The model under review builds one solid part; all positions refer to its coordinate system, in mm. A direction names the side the tool comes from. Give positions to 0.01 mm unless a question says otherwise; leave off trailing zeros. Loops run counter-clockwise (first coordinate to the right, second up) from the corner with the lowest first, then second, coordinate; pieces in that order, holes last. Notation, with made-up numbers: (4, 44) - (25, 44) arc R18 cw to (25, 69) - close; hole circle Ø9 at (74, 1.25). An arc over 180 degrees is marked (long way). Return JSON: item names as keys, results as strings. Group by question number.
from build123d import *

# Parameters (mm, degrees)
SKETCH1_R           = 17.5
SKETCH1_R_2         = 1.5
BOSS_EXTRUDE1_DEPTH = 4
SKETCH3_W           = 12
SKETCH3_H           = 17
SKETCH3_W_2         = 10
SKETCH3_H_2         = 15
BOSS_EXTRUDE2_DEPTH = 10
FILLET1_R           = 2


with BuildPart() as part:
    # Sketch1 → Boss-Extrude1 (new body)
    with BuildSketch(Plane(origin=(0, 0, 0), x_dir=(1, 0, 0), z_dir=(0, 1, 0))):
        with Locations(Location((0, 0, 0), (0, 0, 270))):
            Circle(SKETCH1_R)
        with Locations(Location((12, 6, 0), (0, 0, 270))):
            Circle(SKETCH1_R_2, mode=Mode.SUBTRACT)
        with Locations(Location((12, -6, 0), (0, 0, 270))):
            Circle(SKETCH1_R_2, mode=Mode.SUBTRACT)
        with Locations(Location((-12, 6, 0), (0, 0, 270))):
            Circle(SKETCH1_R_2, mode=Mode.SUBTRACT)
        with Locations(Location((-12, -6, 0), (0, 0, 270))):
            Circle(SKETCH1_R_2, mode=Mode.SUBTRACT)
        with Locations(Location((6, 12, 0), (0, 0, 270))):
            Circle(SKETCH1_R_2, mode=Mode.SUBTRACT)
        with Locations(Location((6, -12, 0), (0, 0, 270))):
            Circle(SKETCH1_R_2, mode=Mode.SUBTRACT)
        with Locations(Location((-6, -12, 0), (0, 0, 270))):
            Circle(SKETCH1_R_2, mode=Mode.SUBTRACT)
        with Locations(Location((-6, 12, 0), (0, 0, 270))):
            Circle(SKETCH1_R_2, mode=Mode.SUBTRACT)
    extrude(amount=BOSS_EXTRUDE1_DEPTH)

    # Sketch3 → Boss-Extrude2 (add)
    with BuildSketch(Plane(origin=(0, 4, 0), x_dir=(1, 0, 0), z_dir=(0, 1, 0))):
        Rectangle(SKETCH3_W, SKETCH3_H)
        Rectangle(SKETCH3_W_2, SKETCH3_H_2, mode=Mode.SUBTRACT)
    extrude(amount=BOSS_EXTRUDE2_DEPTH)

    # Fillet1
    fillet1_edges = [part.edges().sort_by_distance(p)[0] for p in [
        (-6, 4, 0),
        (0, 4, 8.5),
        (6, 4, 0),
        (0, 4, -8.5),
    ]]
    fillet(fillet1_edges, radius=FILLET1_R - 0.0001)  # a hair under: the kernel refuses the full size


solid = part.part
Item 1: For L1, parallel to X at y = 8.5, z = 1.5; L2, parallel to X at y = 2.2, z = 6; L3, parallel to X at y = 1, z = -12, list the stretches that pass through material, from the lowest coordinate up. Write a range as from..to.
Item 2: Take a section at B-B (x = 7). State the section outline as (y, z) points.
Item 3: Mouldability with a two-part tool opening along X and no side actions: class faces 6 (the face through (0, 0, 0)), 7 (the face through (12.07, 1.97, 4.5)), 8 (the face through (-10.648, 1.972, -13.887)) as +X half, -X half, draft (parallel to the pull), parting line (faces both ways), or undercut.
Item 4: Take a section at C-C (z = -12). State the section outline as (x, y) points.
Item 5: Tool access review of faces 1 (the face through (-5.93, 1.97, -13.5)), 2 (the face through (0, 4, 11)), 3 (the face through (-6, 10, 0)), 4 (the face through (0.11, 4.57, 9.1)), 5 (the face through (6, 10, 0)): name each direction out of +Z, -Z, +X, -X, +Y, -Y from which nothing blocks a thin tool from reaching the whole face with its end or side.
Item 6: For P1, Ø6.5, axis at y = 9, z = -2.5, coming from the -X side; P2, Ø4, axis at x = -12, z = 6, coming from the -Y side; P3, Ø4, axis at y = 7.5, z = -5.5, coming from the +X side; P4, Ø2, axis at x = 7.5, y = 10, coming from the -Z side, all flat-tipped, find the tip position at first contact; note any pin that passes through.
Item 7: Take a section at A-A (y = 12.75). State the section outline as (x, z) points.
Item 8: Take a section at D-D (x = 0). State the section outline as (y, z) points, then the cut area to 3 significant figures.
Check sheet entries:
{
 "1": {"L1": "x = -6..-5, 5..6", "L2": "x = -16.44..-13.5, -10.5..10.5, 13.5..16.44", "L3": "x = -12.74..-7.5, -4.5..4.5, 7.5..12.74"},
 "2": {"outline": "(0, -16.04) - (4, -16.04) - (4, -13.12) - (0, -13.12) - close; (0, -10.88) - (4, -10.88) - (4, -10.5) arc R2 cw to (4.27, -9.5) - (4.27, 9.5) arc R2 cw to (4, 10.5) - (4, 10.88) - (0, 10.88) - close; (0, 13.12) - (4, 13.12) - (4, 16.04) - (0, 16.04) - close"},
 "3": {"face 6": "draft", "face 7": "undercut", "face 8": "parting line"},
 "4": {"outline": "(-12.74, 0) - (-7.5, 0) - (-7.5, 4) - (-12.74, 4) - close; (-4.5, 0) - (4.5, 0) - (4.5, 4) - (-4.5, 4) - close; (7.5, 0) - (12.74, 0) - (12.74, 4) - (7.5, 4) - close"},
 "5": {"face 1": "+Y, -Y", "face 2": "+Y", "face 3": "+Z, -Z, -X, +Y", "face 4": "+Z, +X, -X, +Y", "face 5": "+Z, -Z, +X, +Y"},
 "6": {"P1": "stops at x = -6.02", "P2": "stops at y = 0", "P3": "stops at x = 6.06", "P4": "passes through"},
 "7": {"outline": "(-6, -8.5) - (6, -8.5) - (6, 8.5) - (-6, 8.5) - close; hole (-5, -7.5) - (5, -7.5) - (5, 7.5) - (-5, 7.5) - close"},
 "8": {"outline": "(0, -17.5) - (4, -17.5) - (4, -10.5) arc R2 cw to (6, -8.5) - (14, -8.5) - (14, -7.5) - (4, -7.5) - (4, 7.5) - (14, 7.5) - (14, 8.5) - (6, 8.5) arc R2 cw to (4, 10.5) - (4, 17.5) - (0, 17.5) - close", "area": "162 mm^2"}
}
